```python
from build123d import *

# Parameters (mm, degrees)
SKETCH2_R            = 3.50000001
BOSS_EXTRUDE1_DEPTH  = 2.500000004
SKETCH3_R            = 1.999999988
BOSS_EXTRUDE2_DEPTH  = 9.99999999
CUT_EXTRUDE1_START   = -8.000000002
CUT_EXTRUDE1_DEPTH   = 8.000000002
SKETCH5_R            = 5.957710945
BOSS_EXTRUDE3_DEPTH  = 1.27
SKETCH6_W            = 10.160000002
SKETCH6_H            = 5.079999996
BOSS_EXTRUDE4_DEPTH  = 2.54
SKETCH7_R            = 0.381
BOSS_EXTRUDE5_DEPTH  = 6.35
SKETCH8_R            = 0.381
BOSS_EXTRUDE6_DEPTH  = 6.35
SKETCH9_R            = 0.381
BOSS_EXTRUDE7_DEPTH  = 6.35
SKETCH10_R           = 0.381
BOSS_EXTRUDE8_DEPTH  = 6.35
SKETCH11_R           = 0.381
BOSS_EXTRUDE9_DEPTH  = 6.35
SKETCH12_R           = 0.381
BOSS_EXTRUDE10_DEPTH = 6.35


with BuildPart() as part:
    # Sketch1 → Revolve1 (revolve)
    with BuildSketch(Plane.XZ, mode=Mode.PRIVATE) as revolve1_sk:
        Polygon((7.62, 66.649999999), (0, 66.649999999), (0, 12.499999994), (12.200000009, 12.499999994), (12.200000009, 60.299999999), (11.565000009, 60.299999999), (11.565000009, 61.569999999), (1.27, 61.569999999), (1.27, 65.379999999), (7.62, 65.379999999), align=None)
    revolve(revolve1_sk.sketch.rotate(Axis((0, 0, 66.649999999), (0, 0, -1)), 180), axis=Axis((0, 0, 66.649999999), (0, 0, -1)))

    # Sketch2 → Boss-Extrude1 (add)
    with BuildSketch(Plane(origin=(0, 0, 12.499999994), x_dir=(-1, 0, 0), z_dir=(0, 0, -1))):
        Circle(SKETCH2_R)
    extrude(amount=BOSS_EXTRUDE1_DEPTH)

    # Sketch3 → Boss-Extrude2 (add)
    with BuildSketch(Plane(origin=(0, 0, 9.99999999), x_dir=(-1, 0, 0), z_dir=(0, 0, -1))):
        Circle(SKETCH3_R)
    extrude(amount=BOSS_EXTRUDE2_DEPTH)

    # Sketch4 → Cut-Extrude1 (cut)
    with BuildSketch(Plane(origin=(0, 0, 0), x_dir=(-1, 0, 0), z_dir=(0, 0, -1)).offset(CUT_EXTRUDE1_START)):
        with BuildLine():
            Line((-0.968245816, 1.749999997), (0.968245816, 1.749999997))
            ThreePointArc((0.968245816, 1.749999997), (0, 1.999999988), (-0.968245816, 1.749999997))
        make_face()
    extrude(amount=CUT_EXTRUDE1_DEPTH, mode=Mode.SUBTRACT)

    # Sketch5 → Boss-Extrude3 (add)
    with BuildSketch(Plane.XY.offset(66.649999999)):
        Circle(SKETCH5_R)
    extrude(amount=BOSS_EXTRUDE3_DEPTH)

    # Sketch6 → Boss-Extrude4 (add)
    with BuildSketch(Plane.XY.offset(61.569999999)):
        with Locations((0, 7.619999999)):
            Rectangle(SKETCH6_W, SKETCH6_H)
    extrude(amount=BOSS_EXTRUDE4_DEPTH)

    # Sketch7 → Boss-Extrude5 (add)
    with BuildSketch(Plane(origin=(0, 10.159999997, 0), x_dir=(-1, 0, 0), z_dir=(0, 1, 0))):
        with Locations(Location((-2.286, 62.839999999, 0), (0, 0, 270))):
            Circle(SKETCH7_R)
    extrude(amount=BOSS_EXTRUDE5_DEPTH)

    # Sketch8 → Boss-Extrude6 (add)
    with BuildSketch(Plane(origin=(0, 10.159999997, 0), x_dir=(-1, 0, 0), z_dir=(0, 1, 0))):
        with Locations(Location((3.81, 62.839999999, 0), (0, 0, 270))):
            Circle(SKETCH8_R)
    extrude(amount=BOSS_EXTRUDE6_DEPTH)

    # Sketch9 → Boss-Extrude7 (add)
    with BuildSketch(Plane(origin=(0, 10.159999997, 0), x_dir=(-1, 0, 0), z_dir=(0, 1, 0))):
        with Locations(Location((0.762, 62.839999999, 0), (0, 0, 270))):
            Circle(SKETCH9_R)
    extrude(amount=BOSS_EXTRUDE7_DEPTH)

    # Sketch10 → Boss-Extrude8 (add)
    with BuildSketch(Plane(origin=(0, 10.159999997, 0), x_dir=(-1, 0, 0), z_dir=(0, 1, 0))):
        with Locations(Location((2.286, 62.839999999, 0), (0, 0, 270))):
            Circle(SKETCH10_R)
    extrude(amount=BOSS_EXTRUDE8_DEPTH)

    # Sketch11 → Boss-Extrude9 (add)
    with BuildSketch(Plane(origin=(0, 10.159999997, 0), x_dir=(-1, 0, 0), z_dir=(0, 1, 0))):
        with Locations(Location((-0.762, 62.839999999, 0), (0, 0, 270))):
            Circle(SKETCH11_R)
    extrude(amount=BOSS_EXTRUDE9_DEPTH)

    # Sketch12 → Boss-Extrude10 (add)
    with BuildSketch(Plane(origin=(0, 10.159999997, 0), x_dir=(-1, 0, 0), z_dir=(0, 1, 0))):
        with Locations(Location((-3.81, 62.839999999, 0), (0, 0, 270))):
            Circle(SKETCH12_R)
    extrude(amount=BOSS_EXTRUDE10_DEPTH)


solid = part.part
```
Could you check a few things on this model? Use its own coordinates, in mm. A direction names the side the tool comes from. Give positions to 0.01 mm unless a question says otherwise; leave off trailing zeros. Order: outer loops, then holes, each group sorted by start corner. A loop starts at its lowest first (then second) coordinate and runs counter-clockwise, first axis right, second up.
Q1. Suppose I cut it at C-C, the plane y = 0. Write out the boundary of the cut face in (x, z) (3 decimals).
Q2. For faces 1 (the cylindrical face through (0, -2, 5)), 2 (the flat face through (0, 1.75, 4)), 3 (the cylindrical face through (0.992, 7.555, 66.024)), 4 (the flat face through (0, 8, 64.11)), which set-ups out of +Z, -Z, +X, -X, +Y, -Y let a thin tool reach every point of the face, with its end or its side?
Q3. Suppose I cut it at A-A, the plane y = -4.75. Write out the boundary of the cut face in (x, z).
Q4. Suppose I cut it at D-D, the plane z = 49. Write out the boundary of the cut face in (x, y).
Q5. We'd pull the mould along Z, two halves only. Please class faces 5 (the flat face through (0, 0, 0)), 6 (the flat face through (0, 10.16, 63)), 7 (the cylindrical face through (5.683, 1.79, 67.276)): +Z half, -Z half, draft (parallel to the pull), parting line (faces both ways), or undercut.
Q6. I'm going to push flat-ended pins straight in: P1, Ø2, axis at x = -0.5, z = 2.5, coming from the +Y side; P2, Ø1.3, axis at y = 6.5, z = 63, coming from the +X side; P3, Ø4, axis at x = -5, y = 4, coming from the -Z side. Where does each tip first touch, or does it pass through?
Q7. If I drill on line 1 along Z through (x, y) = (3.25, 3.75); line 2 along Z through (x, y) = (2.25, -6.75); line 3 along Z through (x, y) = (6.5, -8.75), over which ranges is the centre line in solid material (lowest first)?
Q8. Suppose I cut it at B-B, the plane x = -10. Write out the boundary of the cut face in (y, z).
Solution:
1. outline: (-12.2, 12.5) - (-3.5, 12.5) - (-3.5, 10) - (-2, 10) - (-2, 0) - (2, 0) - (2, 10) - (3.5, 10) - (3.5, 12.5) - (12.2, 12.5) - (12.2, 60.3) - (11.565, 60.3) - (11.565, 61.57) - (1.27, 61.57) - (1.27, 65.38) - (7.62, 65.38) - (7.62, 66.65) - (5.958, 66.65) - (5.958, 67.92) - (-5.958, 67.92) - (-5.958, 66.65) - (-7.62, 66.65) - (-7.62, 65.38) - (-1.27, 65.38) - (-1.27, 61.57) - (-11.565, 61.57) - (-11.565, 60.3) - (-12.2, 60.3) - close
2. face 1: -Z
2. face 2: -Z, +X, -X, +Y
2. face 3: +Z
2. face 4: +X, -X, +Y
3. outline: (-11.24, 12.5) - (11.24, 12.5) - (11.24, 60.3) - (10.54, 60.3) - (10.54, 61.57) - (-10.54, 61.57) - (-10.54, 60.3) - (-11.24, 60.3) - close; (-5.96, 65.38) - (5.96, 65.38) - (5.96, 66.65) - (3.6, 66.65) - (3.6, 67.92) - (-3.6, 67.92) - (-3.6, 66.65) - (-5.96, 66.65) - close
4. outline: circle Ø24.4 at (0, 0)
5. face 5: -Z half
5. face 6: undercut
5. face 7: draft
6. P1: stops at y = 1.75
6. P2: stops at x = 5.08
6. P3: stops at z = 12.5
7. line 1: z = 12.5 to 61.57, 65.38 to 67.92
7. line 2: z = 12.5 to 61.57, 65.38 to 66.65
7. line 3: z = 12.5 to 61.57
8. outline: (-6.99, 12.5) - (6.99, 12.5) - (6.99, 60.3) - (5.81, 60.3) - (5.81, 61.57) - (-5.81, 61.57) - (-5.81, 60.3) - (-6.99, 60.3) - close
